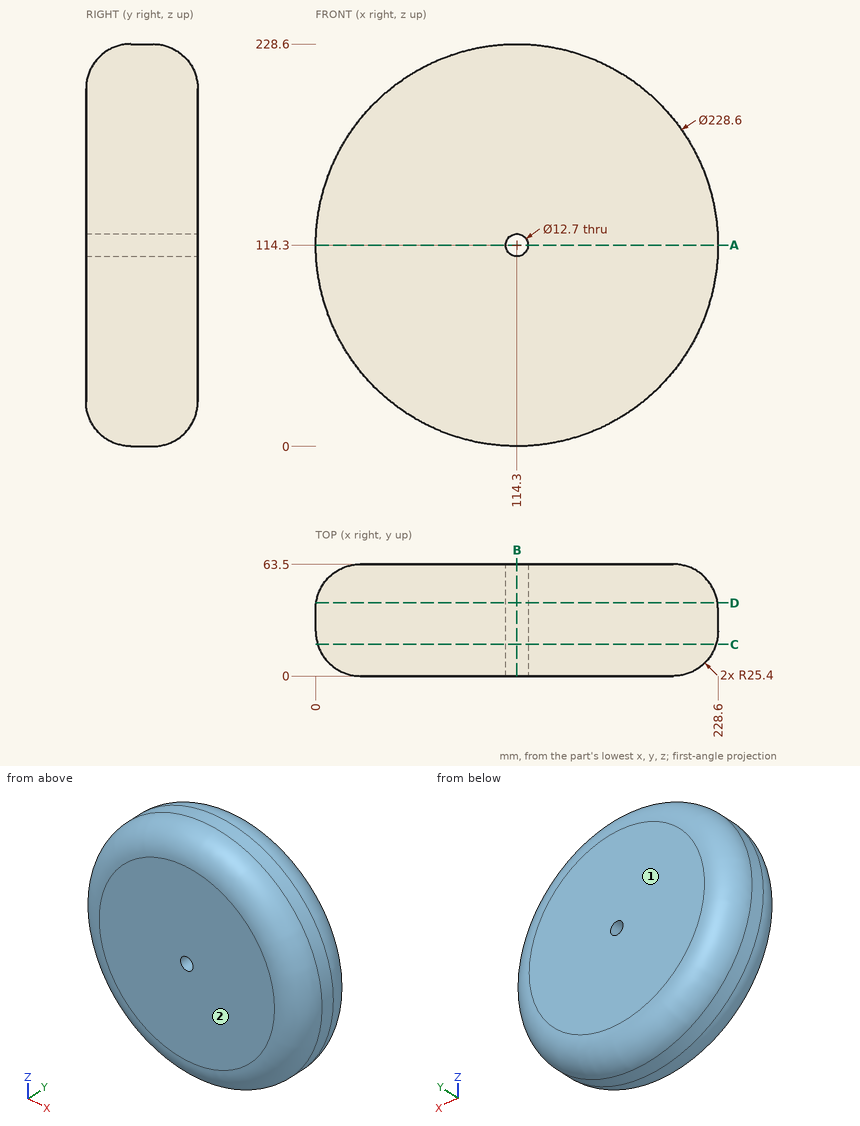
Verification items for this drawing (mm, ordinates from the low corner). Coordinates: 2 decimals unless noted, no trailing zeros. Order: outer loops, then holes, each group sorted by start corner. A loop starts at its lowest first (then second) coordinate and runs counter-clockwise, first axis right, second up. Notation, with made-up numbers: (31, 70) - (67, 70) arc R11 cw to (67, 80) - close; hole circle Ø5 at (62, 65.25). An arc over 180 degrees is marked (long way). Answer as a JSON object with one key per item and string values. Group by question number.
Item 1: Sectioned sample at A-A, the plane z = 114.3. Record the cut outline in (x, y), and give its area (3 significant figures).
Item 2: Scan lines: probe 1 along Z at (x, y) = (114, 37); probe 2 along X at (y, z) = (29, 114.3); probe 3 along X at (y, z) = (43, 114.3). Record each from-to range of solid material in increasing order.
Item 3: Depth check by flat-ended pin: pin 1 Ø10 at (y, z) = (41.5, 200.5) entering from -X; pin 2 Ø16.5 at (x, z) = (114.3, 114.3) entering from -Y; pin 3 Ø2 at (y, z) = (30, 61.5) entering from +X; pin 4 Ø3 at (x, y) = (177, 7.5) entering from -Z. Enter the tip coordinate at first touch or a pass-through.
Item 4: Sectioned sample at D-D, the plane y = 41.5. Record the cut outline in (x, z), and give its area (3 significant figures).
Item 5: Sectioned sample at C-C, the plane y = 18. Record the cut outline in (x, z).
Item 6: Sectioned sample at B-B, the plane x = 114.3. Record the cut outline in (y, z), and give its area (3 significant figures).
Item 7: Draft check along Y on the marked faces 1 and 2. Enter one of: +Y half, -Y half, draft (parallel to the pull), parting line (faces both ways), or undercut.
Resolved:
{
 "1": {"outline": "(0, 25.4) arc R25.4 ccw to (25.4, 0) - (107.95, 0) - (107.95, 63.5) - (25.4, 63.5) arc R25.4 ccw to (0, 38.1) - close; (120.65, 0) - (203.2, 0) arc R25.4 ccw to (228.6, 25.4) - (228.6, 38.1) arc R25.4 ccw to (203.2, 63.5) - (120.65, 63.5) - close", "area": "13,200 mm^2"},
 "2": {"probe 1": "0 to 107.96, 120.64 to 228.6", "probe 2": "0 to 107.95, 120.65 to 228.6", "probe 3": "0.48 to 107.95, 120.65 to 228.12"},
 "3": {"pin 1": "x = 34.11", "pin 2": "y = 0", "pin 3": "x = 216.19", "pin 4": "z = 25.68"},
 "4": {"outline": "circle Ø228.14 at (114.3, 114.3); hole circle Ø12.7 at (114.3, 114.3)", "area": "40,800 mm^2"},
 "5": {"outline": "circle Ø226.4 at (114.3, 114.3); hole circle Ø12.7 at (114.3, 114.3)"},
 "6": {"outline": "(0, 25.4) arc R25.4 ccw to (25.4, 0) - (38.1, 0) arc R25.4 ccw to (63.5, 25.4) - (63.5, 107.95) - (0, 107.95) - close; (0, 120.65) - (63.5, 120.65) - (63.5, 203.2) arc R25.4 ccw to (38.1, 228.6) - (25.4, 228.6) arc R25.4 ccw to (0, 203.2) - close", "area": "13,200 mm^2"},
 "7": {"face 1": "+Y half", "face 2": "-Y half"}
}
